Could you check a few things on this model? Use its own coordinates, in mm. Round coordinates to 2 decimals unless told otherwise and drop trailing zeros. Write each loop counter-clockwise with the first axis right and the second up, starting at its lowest first coordinate (ties: lowest second). Pieces come first, ordered by that corner, then holes. Notation, with made-up numbers: (14, 3) - (42, 3) arc R20 cw to (42, 36) - close; hole circle Ø2 at (70.5, 31). An arc over 180 degrees is marked (long way). Write each question's results on one line, items separated by ' | '. Start each with the question number.
(1) Imagine slicing it at B-B on z = 129.5. Write out the boundary of the cut face in (x, y), then the cut area to 3 significant figures.
(2) Imagine slicing it at D-D on z = 101.5. Write out the boundary of the cut face in (x, y).
(3) Please list where these lines run through material, in increasing order: line 1 (Z direction, x = -56.5, y = 2.35); line 2 (Z direction, x = -61.5, y = 3.15); line 3 (X direction, y = 3.7, z = 161). Write a range as [from, to].
(4) Imagine slicing it at A-A on x = -15. Write out the boundary of the cut face in (y, z), then the cut area to 3 significant figures.
(5) Imagine slicing it at C-C on y = 2.4. State how many separate pieces and enclosed holes the cut face has, then the cut area to 3 significant figures.
(6) For P1, Ø3.5, axis at x = -56.15, z = 161.95, coming from the -Y side; P2, Ø2.5, axis at x = -10, z = 140.75, coming from the +Y side; P3, Ø1.5, axis at x = -14.5, y = 2.5, coming from the +Z side; P4, Ø1.2, axis at y = 1.5, z = 130, coming from the -X side, each with a flat end and sliding along its axis, tell me the tip position at first contact or that it passes through.
```python
from build123d import *

# Parameters (mm, degrees)
BOSS_EXTRUDE1_DEPTH     = 4
SKETCH2_R               = 2.45
SKETCH2_R_2             = 1.5
SKETCH2_W               = 41
SKETCH2_H               = 21
SKETCH2_W_2             = 8.5
SKETCH2_H_2             = 13.5
CUT_EXTRUDE1_DEPTH      = 1
CUT_EXTRUDE1_DEPTH_BACK = 5
CUT_EXTRUDE2_DEPTH      = 1
CUT_EXTRUDE2_DEPTH_BACK = 5
FILLET1_R               = 10
FILLET2_R               = 5


with BuildPart() as part:
    # Sketch1 → Boss-Extrude1 (new body)
    with BuildSketch(Plane(origin=(0, 0, 0), x_dir=(1, 0, 0), z_dir=(0, 1, 0))):
        with BuildLine():
            Line((-120, 0), (-135, 0))
            ThreePointArc((-135, 0), (-138.535533906, -1.464466094), (-140, -5))
            Line((-140, -5), (-140, -20))
            Line((-140, -20), (-140, -178))
            ThreePointArc((-140, -178), (-134.142135624, -192.142135624), (-120, -198))
            Line((-120, -198), (-20, -198))
            ThreePointArc((-20, -198), (-5.857864376, -192.142135624), (0, -178))
            Line((0, -178), (0, -20))
            Line((0, -20), (0, -5))
            ThreePointArc((0, -5), (-1.464466094, -1.464466094), (-5, 0))
            Line((-5, 0), (-20, 0))
            Line((-20, 0), (-120, 0))
        make_face()
    extrude(amount=BOSS_EXTRUDE1_DEPTH)

    # Sketch2 → Cut-Extrude1 (cut, two sides)
    with BuildSketch(Plane(origin=(0, 4, 0), x_dir=(1, 0, 0), z_dir=(0, 1, 0))) as cut_extrude1_sk:
        with Locations((-6.5, -6.5)):
            Circle(SKETCH2_R)
        with Locations((-6.5, -48.5)):
            Circle(SKETCH2_R)
        with Locations((-133.5, -48.5)):
            Circle(SKETCH2_R)
        with Locations((-133.5, -6.5)):
            Circle(SKETCH2_R)
        with Locations((-130, -140.75)):
            Circle(SKETCH2_R_2)
        with Locations((-130, -154.25)):
            Circle(SKETCH2_R_2)
        with Locations((-10, -154.25)):
            Circle(SKETCH2_R_2)
        with Locations((-10, -140.75)):
            Circle(SKETCH2_R_2)
        with Locations((-69.414803196, -44.13296789)):
            Circle(SKETCH2_R_2)
        with Locations((-104.151064992, -151.948209631)):
            Circle(SKETCH2_R_2)
        with Locations((-104.151064992, -161.948209631)):
            Circle(SKETCH2_R_2)
        with Locations((-56.151064992, -161.948209631)):
            Circle(SKETCH2_R_2)
        with Locations((-54.414803196, -44.13296789)):
            Circle(SKETCH2_R_2)
        with Locations((-54.414803196, -61.13296789)):
            Circle(SKETCH2_R_2)
        with Locations((-69.414803196, -61.13296789)):
            Circle(SKETCH2_R_2)
        with Locations((-51.500110177, -90.016074618)):
            Circle(SKETCH2_R_2)
        with Locations((-51.500110177, -141.948209631)):
            Circle(SKETCH2_R_2)
        with Locations((-56.151064992, -151.948209631)):
            Circle(SKETCH2_R_2)
        with Locations((-92.500110177, -141.948209631)):
            Circle(SKETCH2_R_2)
        with Locations((-92.500110177, -90.016074618)):
            Circle(SKETCH2_R_2)
        with Locations((-45.5, -61.5)):
            Circle(SKETCH2_R_2)
        with Locations((-45.5, -3.5)):
            Circle(SKETCH2_R_2)
        with Locations((-94.5, -3.5)):
            Circle(SKETCH2_R_2)
        with Locations((-94.5, -61.5)):
            Circle(SKETCH2_R_2)
        with Locations((-111.497219826, -3.864602307)):
            Circle(SKETCH2_R_2)
        with Locations((-111.497219826, -61.864602307)):
            Circle(SKETCH2_R_2)
        with Locations((-134.497219826, -61.864602307)):
            Circle(SKETCH2_R_2)
        with Locations((-34.958630408, -166.730986033)):
            Circle(SKETCH2_R_2)
        with BuildLine():
            Line((-110.626547642, -161.5), (-110.626547642, -193.5))
            ThreePointArc((-110.626547642, -193.5), (-112.376547642, -195.25), (-114.126547642, -193.5))
            Line((-114.126547642, -193.5), (-114.126547642, -161.5))
            ThreePointArc((-114.126547642, -161.5), (-112.376547642, -159.75), (-110.626547642, -161.5))
        make_face()
        with Locations((-79.990616651, -157.105574446)):
            Rectangle(SKETCH2_W, SKETCH2_H)
        with Locations((-96.791094648, -128.818094274)):
            Rectangle(SKETCH2_W_2, SKETCH2_H_2)
        with BuildLine():
            Line((-46.25, -161.5), (-46.25, -193.5))
            ThreePointArc((-46.25, -193.5), (-48, -195.25), (-49.75, -193.5))
            Line((-49.75, -193.5), (-49.75, -161.5))
            ThreePointArc((-49.75, -161.5), (-48, -159.75), (-46.25, -161.5))
        make_face()
    extrude(amount=CUT_EXTRUDE1_DEPTH, mode=Mode.SUBTRACT)
    extrude(cut_extrude1_sk.sketch, amount=-CUT_EXTRUDE1_DEPTH_BACK, mode=Mode.SUBTRACT)

    # Sketch3 → Cut-Extrude2 (cut, two sides)
    with BuildSketch(Plane(origin=(0, 0, 0), x_dir=(-1, 0, 0), z_dir=(0, -1, 0))) as cut_extrude2_sk:
        with BuildLine():
            Line((0, -65), (28.208630408, -65))
            ThreePointArc((28.208630408, -65), (33.396116586, -66.450731777), (37.078472556, -70.382002569))
            ThreePointArc((37.078472556, -70.382002569), (40.706583622, -72.737954213), (38.208630408, -76.269799027))
            Line((38.208630408, -76.269799027), (38.208630408, -115))
            ThreePointArc((38.208630408, -115), (35.27969822, -122.071067812), (28.208630408, -125))
            Line((28.208630408, -125), (0, -125))
            Line((0, -125), (0, -65))
        make_face()
        with BuildLine():
            Line((140, -65), (140, -125))
            Line((140, -125), (111.791369592, -125))
            ThreePointArc((111.791369592, -125), (104.72030178, -122.071067812), (101.791369592, -115))
            Line((101.791369592, -115), (101.791369592, -76.269799027))
            ThreePointArc((101.791369592, -76.269799027), (99.527050592, -72.782800115), (102.921527444, -70.382002569))
            ThreePointArc((102.921527444, -70.382002569), (106.603883414, -66.450731777), (111.791369592, -65))
            Line((111.791369592, -65), (140, -65))
        make_face()
    extrude(amount=CUT_EXTRUDE2_DEPTH, mode=Mode.SUBTRACT)
    extrude(cut_extrude2_sk.sketch, amount=-CUT_EXTRUDE2_DEPTH_BACK, mode=Mode.SUBTRACT)

    # Fillet1
    fillet1_edges = [part.edges().sort_by_distance(p)[0] for p in [
        (0, 2, 125),
        (-140, 2, 125),
    ]]
    fillet(fillet1_edges, radius=FILLET1_R)

    # Fillet2
    fillet2_edges = [part.edges().sort_by_distance(p)[0] for p in [
        (-140, 2, 65),
        (0, 2, 65),
    ]]
    fillet(fillet2_edges, radius=FILLET2_R)


solid = part.part
```
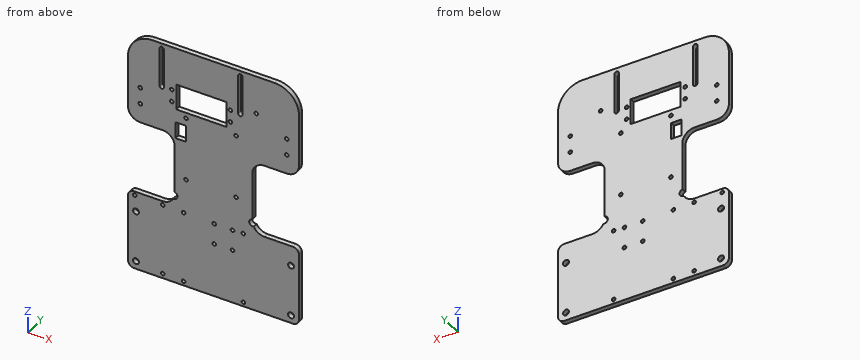
Response:
1) outline: (-138.35, 0) - (-101.04, 0) - (-101.04, 4) - (-138.35, 4) - close; (-92.54, 0) - (-1.65, 0) - (-1.65, 4) - (-92.54, 4) - close | area: 513 mm²
2) outline: (-101.79, 0) - (-38.21, 0) - (-38.21, 4) - (-101.79, 4) - close
3) line 1: [0, 150.49], [153.41, 160.49], [163.41, 198] | line 2: [0, 146.61], [167.61, 198] | line 3: [-140, -114.05], [-110.7, -105.31], [-102.99, -100.49], [-59.49, -57.31], [-54.99, -49.68], [-46.32, 0]
4) outline: (0, 0) - (4, 0) - (4, 65) - (0, 65) - close; (0, 125) - (4, 125) - (4, 197.36) - (0, 197.36) - close | area: 549 mm²
5) separate pieces: 1 | enclosed holes: 32 | area: 21,500 mm²
6) P1: y = 0 | P2: through | P3: z = 197.43 | P4: x = -138.98
